Check sheet for the modelled part. Datum: model origin and axes. Units: mm. Give positions to 0.01 mm unless a question says otherwise; leave off trailing zeros. Order: outer loops, then holes, each group sorted by start corner. A loop starts at its lowest first (then second) coordinate and runs counter-clockwise, first axis right, second up.
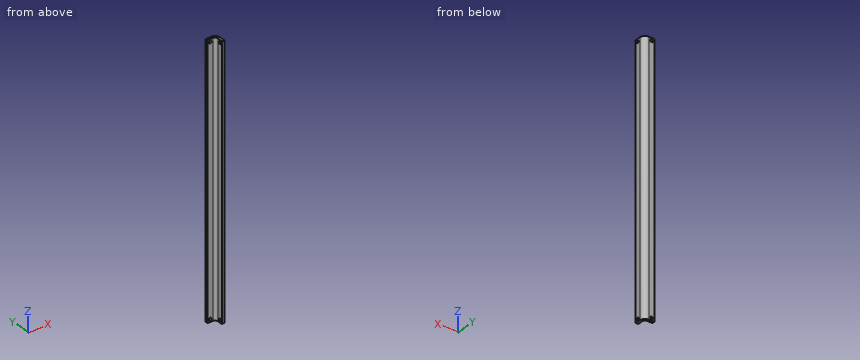
```python
from build123d import *

# Parameters (mm, degrees)
F1_DEPTH = 378.451567
F2_R     = 3.96748
F3_R     = 7.38632
F4_R     = 1.8288
F5_DEPTH = 3.41884
F6_R     = 1.8288
F7_DEPTH = 3.41884
F8_R     = 0.762


with BuildPart() as f1:
    # F0 (on Top) → F1 (new body)
    with BuildSketch(Plane.XY):
        Polygon((-11.90498, 0), (0, 0), (0, -11.90498), (3.41884, -11.90498), (3.41884, 3.41884), (-11.90498, 3.41884), align=None)
    extrude(amount=F1_DEPTH)

    # F2
    f2_edges = [f1.edges().sort_by_distance(p)[0] for p in [
        (0, 0, 189.225784),
    ]]
    fillet(f2_edges, radius=F2_R)

    # F3
    f3_edges = [f1.edges().sort_by_distance(p)[0] for p in [
        (3.41884, 3.41884, 189.225784),
    ]]
    fillet(f3_edges, radius=F3_R)

    # F4 (on face) → F5 (cut, through all)
    with BuildSketch(Plane(origin=(0, 3.41884, 0), x_dir=(-1, 0, 0), z_dir=(0, 1, 0))):
        with Locations((7.93623, 3.96875)):
            Circle(F4_R)
        with Locations((7.93623, 374.482817)):
            Circle(F4_R)
    extrude(amount=-F5_DEPTH, mode=Mode.SUBTRACT)

    # F6 (on face) → F7 (cut, through all)
    with BuildSketch(Plane.YZ.offset(3.41884)):
        with Locations((-7.93623, 374.482817)):
            Circle(F6_R)
        with Locations((-7.93623, 3.96875)):
            Circle(F6_R)
    extrude(amount=-F7_DEPTH, mode=Mode.SUBTRACT)

    # F8
    f8_edges = [f1.edges().sort_by_distance(p)[0] for p in [
        (-11.90498, 1.70942, 378.451567),
        (1.70942, -11.90498, 378.451567),
        (1.70942, -11.90498, 0),
        (-11.90498, 1.70942, 0),
    ]]
    fillet(f8_edges, radius=F8_R)


solid = f1.part
```
(1) Cross-section at A-A on z = 347.5. Enter the section's corners in (x, y).
Response values:
outline: (-11.9, 0) - (-3.97, 0) arc R3.97 cw to (0, -3.97) - (0, -11.9) - (3.42, -11.9) - (3.42, -3.97) arc R7.39 ccw to (-3.97, 3.42) - (-11.9, 3.42) - close
(2) Material ranges on L1, parallel to Z at x = -8.25, y = 2.25; L2, parallel to Z at x = 2, y = -6.5; L3, parallel to Y at x = -4.25, z = 326.5, recorded low to high.
Response values:
L1: z = 0 to 2.17, 5.77 to 372.68, 376.28 to 378.45
L2: z = 0 to 2.84, 5.1 to 373.35, 375.61 to 378.45
L3: y = 0 to 3.42
(3) Gauge pin test, flat ends, axial feed: pin 1 Ø1.5 at (y, z) = (-2, 93.5) entering from -X; pin 2 Ø3 at (x, z) = (-7.94, 3.97) entering from -Y; pin 3 Ø4 at (x, z) = (-6.5, 105.5) entering from -Y; pin 4 Ø5 at (y, z) = (-1, 64.5) entering from +X. Record the tip position at first contact, or that the pin passes through.
Response values:
pin 1: stops at x = -1.08
pin 2: passes through
pin 3: stops at y = 0
pin 4: stops at x = 3.4
